Autodesk Inventor part; units mm, degrees
ref_plane "YZ Plane" through (0, 0, 0) normal (1, 0, 0) x (0, 1, 0)
ref_plane "XZ Plane" through (0, 0, 0) normal (0, 1, 0) x (-1, 0, 0)
sketch "Esboço1" plane through (0, 0, 0) normal (0, 1, 0) x (-1, 0, 0)
  line L0 (25, 30) -> (-25, 30)
  line L1 (-25, 30) -> (-25, -30)
  line L2 (-25, -30) -> (25, -30)
  line L3 (25, -30) -> (25, 30)
  line L4 (25, 30) -> (-25, -30) construction
  line L5 (-25, 30) -> (25, -30) construction
  point P0 (0, 0)
  dimension "d0" = 50
  dimension "d1" = 60
extrude "Extrusão1" add sketch "Esboço1" along normal blind 60
sketch "Esboço2" plane through (25, 0, 30) normal (1, 0, 0) x (0, 0, -1)
  line L0 (0, 60) -> (15, 60)
  line L1 (15, 60) -> (15, 28.9851)
  line L2 (15, 28.9851) -> (0, 28.9851)
  line L3 (0, 28.9851) -> (0, 60)
  line L4 (0, 60) -> (60, 60)
  line L5 (60, 60) -> (45, 60)
  line L6 (45, 60) -> (45, 28.9851)
  line L7 (45, 28.9851) -> (60, 28.9851)
  line L8 (60, 28.9851) -> (60, 60)
  point P0 (30, 0)
  dimension "d4" = 15
  dimension "d5" = 15
extrude "Extrusão2" cut sketch "Esboço2" against normal blind 60
fillet "Arredondamento1" radius 15 2 edges at (0, 60, 15) (0, 60, -15)
sketch "Esboço3" plane through (25, 0, 30) normal (1, 0, 0) x (0, 0, -1)
  arc A0 (45, 45) -> (15, 45) centre (30, 45) ccw
  point P0 (30, 0)
hole "Furo1" at (25, 45, 0) direction (-1, 0, 0) diameter 15 end through all
sketch "Esboço4" plane through (25, 28.9851, 30) normal (0, 1, 0) x (1, 0, 0)
  line L0 (0, 0) -> (-50, 0)
  line L1 (-50, 0) -> (-29.7763, 0)
  line L2 (-21.1397, 5.3332) -> (-6.6144, 5.3332)
  line L3 (-6.6144, 5.3332) -> (0, 0)
  line L4 (0, 0) -> (-34.3564, 0)
  line L5 (-21.1397, 5.3332) -> (-29.7763, 0)
  point P0 (-25, 30)
extrude "Extrusão3" cut sketch "Esboço4" against normal blind 60
mirror "Espelhar1" about plane through (0, 0, 0) normal (0, 0, 1) of "Extrusão3"
Can you work these out from the model? Positions are in its coordinate system, mm. A direction names the side the tool comes from. Give positions to 0.01 mm unless a question says otherwise; leave off trailing zeros. Order: outer loops, then holes, each group sorted by start corner. A loop starts at its lowest first (then second) coordinate and runs counter-clockwise, first axis right, second up. Notation, with made-up numbers: M 36,68.5 L 71,68.5 A11 cw 71,75.5 Z; hole C 5,8.5 d7. An arc over 180 degrees is marked long. Use one line per item in the form item = value. Start each with the question number.
Item 1: If we section it at C-C (z = -4.5): Write out the boundary of the cut face in (x, y).
Item 2: For faces 4 (the flat face through (11, 15, 24.667)), 5 (the flat face through (25, 23, 0)), 6 (the flat face through (11, 15, -24.667)), 7 (the flat face through (0, 28.985, 21)), 8 (the flat face through (0, 37, -15)), which set-ups out of +Z, -Z, +X, -X, +Y, -Y let a thin tool reach every point of the face, with its end or its side?
Item 3: Will these pins go through, and if not, where does the flat tip stop? pin 1 Ø7.5 at (x, y) = (11, 20) entering from -Z; pin 2 Ø13 at (x, y) = (-6.5, 38.5) entering from +Z; pin 3 Ø4.5 at (x, z) = (-5, -26) entering from +Y.
Item 4: If I drill on line 1 along Y through (x, z) = (-8, 0); line 2 along Z through (x, y) = (-7, 45); line 3 along Z through (x, y) = (8, 15), over which ranges is the centre line in solid material (lowest first)?
Item 5: If we section it at D-D (y = 16.5): Write out the boundary of the cut face in (x, z).
Item 6: If we section it at A-A (y = 38.5): Write out the boundary of the cut face in (x, z), then the cut area to 3 significant figures.
Item 7: We'd pull the mould along Z, two halves only. Please class faces 1 (the flat face through (-25, 23, 0)), 2 (the flat face through (0, 37, 15)), 3 (the cylindrical face through (-0.35, 52.32, 1.63)): +Z half, -Z half, draft (parallel to the pull), parting line (faces both ways), or undercut.
Outcome:
q1.outline = M -25,0 L 25,0 L 25,39 L -25,39 Z; M -25,51 L 25,51 L 25,59.31 L -25,59.31 Z
q2.face_4 = +Z, +Y, -Y
q2.face_5 = +Z, -Z, +X, +Y, -Y
q2.face_6 = -Z, +Y, -Y
q2.face_7 = +Z, +X, -X, +Y
q2.face_8 = -Z, +X, -X, +Y
q3.pin_1 = -24.67
q3.pin_2 = 15
q3.pin_3 = 28.99
q4.line_1 = 0 to 37.5, 52.5 to 60
q4.line_2 = -15 to -7.5, 7.5 to 15
q4.line_3 = -24.67 to 24.67
q5.outline = M -25,-30 L -4.78,-30 L 3.86,-24.67 L 18.39,-24.67 L 25,-30 L 25,30 L 18.39,24.67 L 3.86,24.67 L -4.78,30 L -25,30 Z
q6.outline = M -25,-15 L 25,-15 L 25,-3.74 L -25,-3.74 Z; M -25,3.74 L 25,3.74 L 25,15 L -25,15 Z
q6.area = 1,130 mm2
q7.face_1 = draft
q7.face_2 = +Z half
q7.face_3 = undercut
